Design review of the part built by this model. Coordinates are the model's own, in mm. A direction names the side the tool comes from. Coordinates: 2 decimals unless noted, no trailing zeros. Loops run counter-clockwise (first coordinate to the right, second up) from the corner with the lowest first, then second, coordinate; pieces in that order, holes last. Notation, with made-up numbers: (-22.5, 66) - (35.5, 66) arc R16 cw to (35.5, 88) - close; hole circle Ø8 at (29, 89.5). An arc over 180 degrees is marked (long way). Answer in a Markdown table with one row per item. Add a question column.
(1) To check wall thickness, follow L1, parallel to Z at x = -0.75, y = 0.2; L2, parallel to Z at x = 1.2, y = 1.35; L3, parallel to X at y = 1.05, z = 3.75. State the ranges of each line that lie inside material, in increasing order. Write a range as [from, to].
(2) The part is to be moulded in two halves that separate along Y. For faces 1 (the face through (2.61, -0.58, 6.3)), 2 (the face through (0, 0, -9)), 3 (the face through (-0.63, -1.08, 8.19)), say which applies: released by +Y, released by -Y, zero draft, split by the parting line, or undercut.
(3) Clearance check with flat-ended pins moving along their axes: pin 1 (3 mm diameter, centred on x = 2, z = 7, fed in from +Y); pin 2 (3 mm diameter, centred on x = -1.5, y = 0.5, fed in from -Z); pin 3 (1 mm diameter, centred on x = 2, y = 2, fed in from -Z); pin 4 (1.2 mm diameter, centred on x = -0.5, y = 0.5, fed in from +Z). State where each tip first meets the part, or that it passes through.
(4) We need section A-A, the plane z = -4.5. Write out the cut boundary in (x, y), plus the area to 3 significant figures.
(5) For faces 4 (the face through (-0.07, -1.5, -1.51)), 5 (the face through (2, 0, 9)), 6 (the face through (1.25, 0, 8)), list the 3-axis set-ups (+Z, -Z, +X, -X, +Y, -Y) from which the entire face can be reached by the end or side of a thin tool; tool diameter is ignored.
from build123d import *

# Parameters (mm, degrees)
CUT_EXTRUDE1_START = -1.5
CUT_EXTRUDE1_DEPTH = 1.5
SKETCH4_R          = 1.551628848
CUT_EXTRUDE2_DEPTH = 1.5
CUT_EXTRUDE2_TAPER = 45


with BuildPart() as part:
    # Sketch2 → Revolve1 (revolve)
    with BuildSketch(Plane(origin=(0, 0, 0), x_dir=(0, 0, -1), z_dir=(1, 0, 0))):
        with BuildLine():
            Line((-9, 0), (-9, 2.580583739))
            ThreePointArc((-9, 2.580583739), (-8.996431853, 2.598522025), (-8.98627063, 2.61372937))
            Line((-8.98627063, 2.61372937), (-8.86372937, 2.73627063))
            ThreePointArc((-8.86372937, 2.73627063), (-8.848522025, 2.746431853), (-8.830583739, 2.75))
            Line((-8.830583739, 2.75), (-6.656916261, 2.75))
            ThreePointArc((-6.656916261, 2.75), (-6.638977975, 2.746431853), (-6.62377063, 2.73627063))
            Line((-6.62377063, 2.73627063), (-6.57622937, 2.68872937))
            ThreePointArc((-6.57622937, 2.68872937), (-6.561022025, 2.678568147), (-6.543083739, 2.675))
            Line((-6.543083739, 2.675), (-6.06875, 2.675))
            ThreePointArc((-6.06875, 2.675), (-6.020136409, 2.654863591), (-6, 2.60625))
            Line((-6, 2.60625), (-6, 1.65))
            ThreePointArc((-6, 1.65), (-5.956066017, 1.543933983), (-5.85, 1.5))
            Line((-5.85, 1.5), (8.675240474, 1.5))
            Line((8.675240474, 1.5), (9, 1.175240474))
            Line((9, 1.175240474), (9, 0))
            Line((9, 0), (-9, 0))
        make_face()
    revolve(axis=Axis((0, 0, -9), (0, 0, 1)))

    # Sketch3 → Cut-Extrude1 (cut)
    with BuildSketch(Plane.XY.offset(9).offset(CUT_EXTRUDE1_START)):
        Polygon((1.25, -0.721687836), (1.25, 0.721687836), (0, 1.443375673), (-1.25, 0.721687836), (-1.25, -0.721687836), (0, -1.443375673), align=None)
    extrude(amount=CUT_EXTRUDE1_DEPTH, mode=Mode.SUBTRACT)

    # Sketch4 → Cut-Extrude2 (cut)
    with BuildSketch(Plane.XY.offset(9)):
        Circle(SKETCH4_R)
    extrude(amount=-CUT_EXTRUDE2_DEPTH, taper=CUT_EXTRUDE2_TAPER, mode=Mode.SUBTRACT)


solid = part.part
Responses:
| question | item | result |
|---|---|---|
| 1 | L1 | z = [-9, 7.5] |
| 1 | L2 | z = [6, 9] |
| 1 | L3 | x = [-1.07, 1.07] |
| 2 | face 1 | split by the parting line |
| 2 | face 2 | zero draft |
| 2 | face 3 | undercut |
| 3 | pin 1 | stops at y = 2.7 |
| 3 | pin 2 | stops at z = -9 |
| 3 | pin 3 | stops at z = 6 |
| 3 | pin 4 | stops at z = 8.76 |
| 4 | outline | circle Ø3 at (0, 0) |
| 4 | area | 7.07 mm2 |
| 5 | face 4 | -Z |
| 5 | face 5 | +Z, +X, -X, +Y, -Y |
| 5 | face 6 | +Z |
